```python
from build123d import *

# Parameters (mm, degrees)
SKETCH003_R  = 1.5
PAD003_DEPTH = 20
SKETCH002_R  = 1.5
PAD002_DEPTH = 20
SKETCH001_W  = 12
SKETCH001_H  = 10
PAD001_DEPTH = 20
SKETCH_W     = 15
SKETCH_H     = 13
SKETCH_W_2   = 30
SKETCH_H_2   = 10
PAD_DEPTH    = 20


with BuildPart() as body003:
    # Sketch003 → Pad003 (new body)
    with BuildSketch(Plane.XZ):
        with Locations((20, 5)):
            Circle(SKETCH003_R)
    extrude(amount=PAD003_DEPTH)


with BuildPart() as body002:
    # Sketch002 → Pad002 (new body)
    with BuildSketch(Plane.XZ):
        with Locations((-20, 5)):
            Circle(SKETCH002_R)
    extrude(amount=PAD002_DEPTH)


with BuildPart() as body001:
    # Sketch001 → Pad001 (new body)
    with BuildSketch(Plane.XZ):
        with Locations((0, 5)):
            Rectangle(SKETCH001_W, SKETCH001_H)
    extrude(amount=PAD001_DEPTH)


with BuildPart() as cut002:
    # Sketch → Pad (new body)
    with BuildSketch(Plane.XZ):
        with Locations((0, 6.5)):
            Rectangle(SKETCH_W, SKETCH_H)
        with Locations((-22.5, 5)):
            Rectangle(SKETCH_W_2, SKETCH_H_2)
        with Locations((22.5, 5)):
            Rectangle(SKETCH_W_2, SKETCH_H_2)
    extrude(amount=PAD_DEPTH)

    # Cut: cut Body001
    add(body001.part, mode=Mode.SUBTRACT)

    # Cut001: cut Body002
    add(body002.part, mode=Mode.SUBTRACT)

    # Cut002: cut Body003
    add(body003.part, mode=Mode.SUBTRACT)


solid = cut002.part
```
The model under review builds one solid part; all positions refer to its coordinate system, in mm. A direction names the side the tool comes from. Give positions to 0.01 mm unless a question says otherwise; leave off trailing zeros. Loops run counter-clockwise (first coordinate to the right, second up) from the corner with the lowest first, then second, coordinate; pieces in that order, holes last. Notation, with made-up numbers: (77, -9.75) -> (86, -9.75) arc R22 ccw to (86, 19.25) -> close; hole circle Ø9 at (-40, 78). An arc over 180 degrees is marked (long way). Use CSV: the item, a comma, the result in double quotes.
1. Consider section C-C, the plane z = 5. Write out the cut boundary in (x, y).
Result:
outline,"(-37.5, -20) -> (-21.5, -20) -> (-21.5, 0) -> (-37.5, 0) -> close; (-18.5, -20) -> (-6, -20) -> (-6, 0) -> (-18.5, 0) -> close; (6, -20) -> (18.5, -20) -> (18.5, 0) -> (6, 0) -> close; (21.5, -20) -> (37.5, -20) -> (37.5, 0) -> (21.5, 0) -> close"
2. Machinability: for faces 4 (the face through (-23, -10, 10)), 5 (the face through (22, -10, 0)), 6 (the face through (7.5, -10, 11)), 7 (the face through (-37.5, -10, 5)), 8 (the face through (0, -10, 10)), which of the approach directions +Z, -Z, +X, -X, +Y, -Y give a long, thin tool a straight path to every point of the face, cutting with its end or side? Answer none if there is none.
Result:
face 4,"+Z, -X, +Y, -Y"
face 5,"-Z, +X, -X, +Y, -Y"
face 6,"+Z, +X, +Y, -Y"
face 7,"+Z, -Z, -X, +Y, -Y"
face 8,"-Z, +Y, -Y"
3. Consider section D-D, the plane y = -11.5. Write out the cut boundary in (x, z).
Result:
outline,"(-37.5, 0) -> (-6, 0) -> (-6, 10) -> (6, 10) -> (6, 0) -> (37.5, 0) -> (37.5, 10) -> (7.5, 10) -> (7.5, 13) -> (-7.5, 13) -> (-7.5, 10) -> (-37.5, 10) -> close; hole circle Ø3 at (-20, 5); hole circle Ø3 at (20, 5)"
4. The part is to be moulded in two halves that separate along X. For faces 1 (the face through (0, -10, 13)), 2 (the face through (6, -10, 5)), 3 (the face through (-7.5, -10, 11)), say which applies: +X half, -X half, draft (parallel to the pull), parting line (faces both ways), or undercut.
Result:
face 1,"draft"
face 2,"undercut"
face 3,"-X half"
5. For P1, Ø1, axis at x = -5, y = -10.5, coming from the -Z side; P2, Ø2, axis at y = -15, z = 11.5, coming from the +X side; P3, Ø1.5, axis at y = -8.5, z = 11, coming from the -X side, all flat-tipped, find the tip position at first contact; note any pin that passes through.
Result:
P1,"stops at z = 10"
P2,"stops at x = 7.5"
P3,"stops at x = -7.5"
6. Consider section A-A, the plane z = 8. Write out the cut boundary in (x, y), then the cut area to 3 significant figures.
Result:
outline,"(-37.5, -20) -> (-6, -20) -> (-6, 0) -> (-37.5, 0) -> close; (6, -20) -> (37.5, -20) -> (37.5, 0) -> (6, 0) -> close"
area,"1,260 mm²"
7. Consider section B-B, the plane x = -20. Write out the cut boundary in (y, z), then the cut area to 3 significant figures.
Result:
outline,"(-20, 0) -> (0, 0) -> (0, 3.5) -> (-20, 3.5) -> close; (-20, 6.5) -> (0, 6.5) -> (0, 10) -> (-20, 10) -> close"
area,"140 mm²"
8. To check wall thickness, follow probe 1 along X at (y, z) = (-13, 5.25); probe 2 along Z at (x, y) = (20, -10); probe 3 along X at (y, z) = (-12.75, 5.75). State the ranges of each line that lie inside material, in increasing order. Write a range as from..to.
Result:
probe 1,"x = -37.5..-21.48, -18.52..-6, 6..18.52, 21.48..37.5"
probe 2,"z = 0..3.5, 6.5..10"
probe 3,"x = -37.5..-21.3, -18.7..-6, 6..18.7, 21.3..37.5"
